Build history of the part. All positions in model axes, mm. A direction names the side the tool comes from. Round coordinates to 2 decimals unless told otherwise and drop trailing zeros. Order: outer loops, then holes, each group sorted by start corner. A loop starts at its lowest first (then second) coordinate and runs counter-clockwise, first axis right, second up. Notation, with made-up numbers: (33.25, -21.75) -> (90.25, -21.75) arc R31 ccw to (90.25, 13.25) -> close; hole circle Ø8 at (41.5, 7.5). An arc over 180 degrees is marked (long way). Answer as CSV lines item,"result". Start each with the question number.
```python
from build123d import *

# Parameters (mm, degrees)
BOSS_EXTRUDE1_DEPTH = 15
SKETCH3_R           = 26
CUT_EXTRUDE1_DEPTH  = 5
CUT_EXTRUDE2_START  = -5
SKETCH4_R           = 26
CUT_EXTRUDE2_DEPTH  = 5
SKETCH5_R           = 6
BOSS_EXTRUDE2_DEPTH = 8
BOSS_EXTRUDE2_TAPER = 4
SKETCH6_R           = 6
BOSS_EXTRUDE3_DEPTH = 5
SKETCH7_R           = 3.084221082
CUT_EXTRUDE3_DEPTH  = 12
CUT_EXTRUDE4_REACH  = 57.352
SKETCH8_R           = 1


with BuildPart() as part:
    # Sketch1 → Boss-Extrude1 (new body)
    with BuildSketch(Plane.XY):
        with BuildLine():
            Line((-3.570594462, 29.667493479), (-2.97005784, 36.705576615))
            Line((-2.97005784, 36.705576615), (3.376008048, 36.866330498))
            Line((3.376008048, 36.866330498), (3.990261273, 29.667493478))
            ThreePointArc((3.990261273, 29.667493478), (10.470437707, 28.097419204), (16.443765143, 25.134788755))
            Line((16.443765143, 25.134788755), (21.427795521, 30.140255732))
            Line((21.427795521, 30.140255732), (26.392494634, 26.184227828))
            Line((26.392494634, 26.184227828), (22.235716663, 20.274764369))
            ThreePointArc((22.235716663, 20.274764369), (26.190595521, 14.906640576), (28.862087666, 8.797553119))
            Line((28.862087666, 8.797553119), (35.897528594, 9.428290308))
            Line((35.897528594, 9.428290308), (37.157823041, 3.20655004))
            Line((37.157823041, 3.20655004), (30.175016484, 1.351563771))
            ThreePointArc((30.175016484, 1.351563771), (29.754065995, -5.302804758), (27.873701984, -11.699839306))
            Line((27.873701984, -11.699839306), (33.668592462, -15.738960845))
            Line((33.668592462, -15.738960845), (30.634776465, -21.315192059))
            Line((30.634776465, -21.315192059), (24.093274115, -18.247732447))
            ThreePointArc((24.093274115, -18.247732447), (19.493461691, -23.074692722), (13.941084742, -26.766430803))
            Line((13.941084742, -26.766430803), (15.783931113, -33.585461212))
            Line((15.783931113, -33.585461212), (9.875560893, -35.907002814))
            Line((9.875560893, -35.907002814), (6.8362044, -29.352395764))
            ThreePointArc((6.8362044, -29.352395764), (0.209833396, -30.093359427), (-6.416537607, -29.352395762))
            Line((-6.416537607, -29.352395762), (-9.388023643, -35.760634927))
            Line((-9.388023643, -35.760634927), (-15.406355994, -33.741211801))
            Line((-15.406355994, -33.741211801), (-13.521417949, -26.766430798))
            ThreePointArc((-13.521417949, -26.766430798), (-19.073794896, -23.074692716), (-23.673607318, -18.24773244))
            Line((-23.673607318, -18.24773244), (-30.069034419, -21.246694037))
            Line((-30.069034419, -21.246694037), (-33.381284309, -15.831216706))
            Line((-33.381284309, -15.831216706), (-27.454035185, -11.699839298))
            ThreePointArc((-27.454035185, -11.699839298), (-29.334399194, -5.302804748), (-29.755349682, 1.351563781))
            Line((-29.755349682, 1.351563781), (-36.58222643, 3.165127213))
            Line((-36.58222643, 3.165127213), (-35.638555324, 9.442696719))
            Line((-35.638555324, 9.442696719), (-28.442420861, 8.797553128))
            ThreePointArc((-28.442420861, 8.797553128), (-25.770928714, 14.906640584), (-21.816049855, 20.274764376))
            Line((-21.816049855, 20.274764376), (-25.880004748, 26.052266352))
            Line((-25.880004748, 26.052266352), (-21.121966844, 30.254583494))
            Line((-21.121966844, 30.254583494), (-16.024098333, 25.13478876))
            ThreePointArc((-16.024098333, 25.13478876), (-10.050770896, 28.097419207), (-3.570594462, 29.667493479))
        make_face()
    extrude(amount=BOSS_EXTRUDE1_DEPTH)

    # Sketch3 → Cut-Extrude1 (cut)
    with BuildSketch(Plane.XY.offset(15)):
        Circle(SKETCH3_R)
    extrude(amount=-CUT_EXTRUDE1_DEPTH, mode=Mode.SUBTRACT)

    # Sketch4 → Cut-Extrude2 (cut)
    with BuildSketch(Plane(origin=(0, 0, 0), x_dir=(-1, 0, 0), z_dir=(0, 0, -1)).offset(CUT_EXTRUDE2_START)):
        with Locations(Location((0, 0, 0), (0, 0, 180))):
            Circle(SKETCH4_R)
    extrude(amount=CUT_EXTRUDE2_DEPTH, mode=Mode.SUBTRACT)

    # Sketch5 → Boss-Extrude2 (add)
    with BuildSketch(Plane.XY.offset(10)):
        Circle(SKETCH5_R)
    extrude(amount=BOSS_EXTRUDE2_DEPTH, taper=BOSS_EXTRUDE2_TAPER)

    # Sketch6 → Boss-Extrude3 (add)
    with BuildSketch(Plane(origin=(0, 0, 5), x_dir=(-1, 0, 0), z_dir=(0, 0, -1))):
        Circle(SKETCH6_R)
    extrude(amount=BOSS_EXTRUDE3_DEPTH)

    # Sketch7 → Cut-Extrude3 (cut)
    with BuildSketch(Plane.XY.offset(18)):
        Circle(SKETCH7_R)
    extrude(amount=-CUT_EXTRUDE3_DEPTH, mode=Mode.SUBTRACT)

    # Cut-Extrude4: up to this cone (the profile starts inside it)
    cut_extrude4_end = Plane(origin=(0, 0, 15.4184), z_dir=(0, 0, -1)) * Cone(1.182636436, 10.059580688, 126.946217124, mode=Mode.PRIVATE)
    # Sketch8 → Cut-Extrude4 (cut, up to the surface)
    with BuildSketch(Plane(origin=(0, 0, 0), x_dir=(1, 0, 0), z_dir=(0, 1, 0)), mode=Mode.PRIVATE) as cut_extrude4_sk1:
        with Locations(Location((0, -15.418399821, 0), (0, 0, 270))):
            Circle(SKETCH8_R)
    cut_extrude4_tool1 = extrude(cut_extrude4_sk1.sketch, amount=-CUT_EXTRUDE4_REACH, mode=Mode.PRIVATE) & cut_extrude4_end
    add(cut_extrude4_tool1.solids().sort_by_distance((0, 0, 15.4184))[0], mode=Mode.SUBTRACT)


solid = part.part
```
Q1. Slice it at A-A, the plane x = 25. Write the cut outline in (y, z).
Q2. Flat gauge pins, fed straight in: pin 1 Ø3.5 at (x, y) = (0, 0) entering from +Z; pin 2 Ø2.5 at (x, z) = (0, 15.42) entering from +Y; pin 3 Ø2 at (y, z) = (29, 5) entering from +X; pin 4 Ø15.5 at (x, y) = (-5, -8.5) entering from -Z. Where does each tip first touch, or does it go through?
Q3. Probe L1, parallel to Y at x = 0, z = 3.2; L2, parallel to Y at x = 0, z = 13.5; L3, parallel to Y at x = 0, z = 10.5. List the from-to ranges inside material, lowest first.
Q4. Which spindle directions (+Z, -Z, +X, -X, +Y, -Y) get a long thin tool onto all of the face, cutting with end or side? Do faces 1 (the face through (14.85, -30.13, 7.4)), 2 (the face through (0.04, -4.28, 14.42)), 3 (the face through (32.33, 9.11, 7.4)), 4 (the face through (1.66, 2.6, 12.08)), 5 (the face through (-23.82, 23.123, 7.395)). Say none if no direction does.
Q5. Slice it at B-B, the plane z = 2.5. Count the separate pieces of the cut face and the enclosed holes in it, plus the area to 3 significant figures.
Q6. Two-plate mould, pull along Y, no slides. Class faces 6 (the face through (-29.32, -5.39, 7.4)), 7 (the face through (-10.139, 28.065, 7.395)), 8 (the face through (0.303, -30.093, 7.395)): +Y half, -Y half, draft (parallel to the pull), parting line (faces both ways), or undercut.
Q7. Slice it at D-D, the plane x = -7.5. Write the cut outline in (y, z).
Solutions:
1,outline,"(-18.67, 0) -> (-7.14, 0) -> (-7.14, 5) -> (7.14, 5) -> (7.14, 0) -> (16.8, 0) -> (16.8, 15) -> (7.14, 15) -> (7.14, 10) -> (-7.14, 10) -> (-7.14, 15) -> (-18.67, 15) -> close; (24.2, 0) -> (27.29, 0) -> (27.29, 15) -> (24.2, 15) -> close"
2,pin 1,"stops at z = 6"
2,pin 2,"stops at y = 36.81"
2,pin 3,"stops at x = 24.11"
2,pin 4,"stops at z = 0"
3,L1,"y = -30.09 to -26, -6 to 6, 26 to 36.78"
3,L2,"y = -30.09 to -26, -5.76 to -3.08, 3.08 to 5.76, 26 to 36.78"
3,L3,"y = -30.09 to -26, -5.97 to -3.08, 3.08 to 5.97, 26 to 36.78"
4,face 1,"+Z, -Z, +X"
4,face 2,"none"
4,face 3,"+Z, -Z, +Y"
4,face 4,"+Z"
4,face 5,"+Z, -Z, -X"
5,separate pieces,"2"
5,enclosed holes,"1"
5,area,"1,250 mm2"
6,face 6,"undercut"
6,face 7,"+Y half"
6,face 8,"-Y half"
7,outline,"(-31.69, 0) -> (-24.89, 0) -> (-24.89, 5) -> (24.89, 5) -> (24.89, 0) -> (28.9, 0) -> (28.9, 15) -> (24.89, 15) -> (24.89, 10) -> (-24.89, 10) -> (-24.89, 15) -> (-31.69, 15) -> close"
